Build history of the part. All positions in model axes, mm. Face numbers are marked on the shaded views. A direction names the side the tool comes from. Give positions to 0.01 mm unless a question says otherwise; leave off trailing zeros. Order: outer loops, then holes, each group sorted by start corner. A loop starts at its lowest first (then second) coordinate and runs counter-clockwise, first axis right, second up. Notation, with made-up numbers: (59, 62.5) - (64, 62.5) arc R17 ccw to (64, 67.5) - close; hole circle Ø10 at (-3.75, 40). An arc over 180 degrees is marked (long way). Answer in a Markdown table with one row per item.
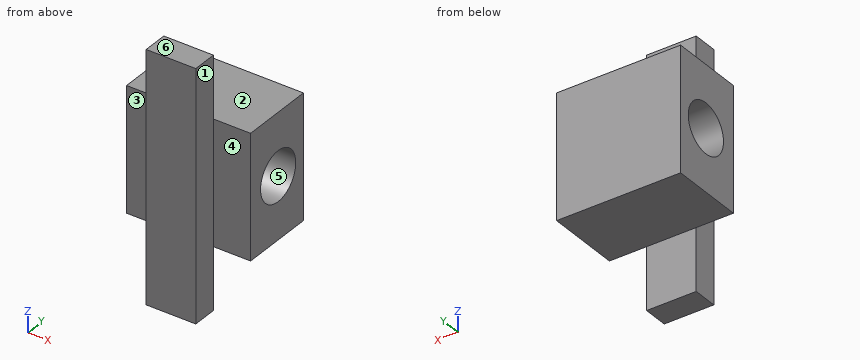
Autodesk Inventor part; units mm, degrees
ref_plane "YZ Plane" through (0, 0, 0) normal (1, 0, 0) x (0, 1, 0)
ref_plane "XZ Plane" through (0, 0, 0) normal (0, 1, 0) x (-1, 0, 0)
ref_plane "XY Plane" through (0, 0, 0) normal (0, 0, 1) x (1, 0, 0)
sketch "Sketch1" plane through (0, 0, 0) normal (0, 1, 0) x (-1, 0, 0)
  line L0 (-10, -50) -> (10, -50)
  line L1 (10, -50) -> (10, 50)
  line L2 (10, 50) -> (-10, 50)
  line L3 (-10, 50) -> (-10, -50)
  line L4 (-10, -50) -> (10, 50) construction
  line L5 (10, -50) -> (-10, 50) construction
  point P0 (0, 0)
  dimension "d0" = 20
  dimension "d1" = 100
extrude "Extrusion1" add sketch "Sketch1" along normal blind 10
sketch "Sketch2" plane through (0, 10, 0) normal (0, 1, 0) x (1, 0, 0)
  line L0 (25, 25) -> (-25, 25)
  line L1 (-25, 25) -> (-25, -25)
  line L2 (-25, -25) -> (25, -25)
  line L3 (25, -25) -> (25, 25)
  line L4 (25, 25) -> (-25, -25) construction
  line L5 (-25, 25) -> (25, -25) construction
  point P0 (0, 0)
  dimension "d4" = 50
  dimension "d5" = 50
extrude "Extrusion2" add sketch "Sketch2" along normal blind 30
sketch "Sketch3" plane through (-25, 10, -25) normal (-1, 0, 0) x (0, 0, 1)
  circle A0 centre (25, 15.6421) radius 10
  point P0 (25, -10)
  dimension "d8" = 20
extrude "Extrusion3" cut sketch "Sketch3" against normal through all
1. Cut at C-C on y = 31. Write the cut outline in (x, z).
Check result:
| item | result |
|---|---|
| outline | (-25, -25) - (25, -25) - (25, -8.44) - (-25, -8.44) - close; (-25, 8.44) - (25, 8.44) - (25, 25) - (-25, 25) - close |
2. Which spindle directions (+Z, -Z, +X, -X, +Y, -Y) get a long thin tool onto all of the face, cutting with end or side? Do the marked faces 1, 2 and 3. Say none if no direction does.
Check result:
| item | result |
|---|---|
| face 1 | +Z, -Z, +X, -Y |
| face 2 | +Z, +X, -X, +Y |
| face 3 | +Z, -Z, -X, -Y |
3. Cut at B-B on y = 20. Write the cut outline in (x, z).
Check result:
| item | result |
|---|---|
| outline | (-25, -25) - (25, -25) - (25, -8.26) - (-25, -8.26) - close; (-25, 8.26) - (25, 8.26) - (25, 25) - (-25, 25) - close |
4. Cut at D-D on x = -21. Write the cut outline in (y, z).
Check result:
| item | result |
|---|---|
| outline | (10, -25) - (40, -25) - (40, 25) - (10, 25) - close; hole circle Ø20 at (25.64, 0) |
5. Probe line 1 (Y direction, x = 5, z = 0); line 2 (Y direction, x = -13, z = 0); line 3 (Y direction, x = 1, z = -35). List the from-to ranges inside material, lowest first.
Check result:
| item | result |
|---|---|
| line 1 | y = 0 to 15.64, 35.64 to 40 |
| line 2 | y = 10 to 15.64, 35.64 to 40 |
| line 3 | y = 0 to 10 |
6. Cut at A-A on z = 0. Write the cut outline in (x, y).
Check result:
| item | result |
|---|---|
| outline | (-25, 10) - (-10, 10) - (-10, 0) - (10, 0) - (10, 10) - (25, 10) - (25, 15.64) - (-25, 15.64) - close; (-25, 35.64) - (25, 35.64) - (25, 40) - (-25, 40) - close |
7. Drop flat-ended pins along their axis: P1, Ø3, axis at x = -10.5, z = 25.5, coming from the -Y side; P2, Ø6, axis at x = 3.5, z = 42, coming from the +Y side; P3, Ø7.5, axis at x = -17, z = -10, coming from the -Y side; P4, Ø5, axis at x = -14.5, y = 34, coming from the +Z side. Give the stop position or say it passes through.
Check result:
| item | result |
|---|---|
| P1 | stops at y = 0 |
| P2 | stops at y = 10 |
| P3 | stops at y = 10 |
| P4 | stops at z = 25 |
8. Two-plate mould, pull along Z, no slides. Class the marked faces 4, 5 and 6: +Z half, -Z half, draft (parallel to the pull), parting line (faces both ways), or undercut.
Check result:
| item | result |
|---|---|
| face 4 | draft |
| face 5 | undercut |
| face 6 | +Z half |
